Input: part model. Units: mm. Frame: model coordinates. Round coordinates to 2 decimals unless told otherwise and drop trailing zeros. Loops run counter-clockwise (first coordinate to the right, second up) from the corner with the lowest first, then second, coordinate; pieces in that order, holes last. Notation, with made-up numbers: M -33,16 L 8,16 A15 ccw 8,25 Z; hole C -4,69 d4. An arc over 180 degrees is marked long. Put each result on its own line as item: value. Start each with the question number.
1) Section B-B on z = 0.25. State how many separate pieces and enclosed holes the cut face has, plus the area to 3 significant figures.
2) Line query: probe 1 along X at (y, z) = (-4.75, 1.2); probe 2 along X at (y, z) = (-6.25, 0.3); probe 3 along Y at (x, z) = (18, 0.9) (3 decimals). Output: solid intervals per line, ascending.
3) Section A-A on y = 5.5. Output: boundary loops of the cut face in (x, z), plus the area to 3 significant figures.
4) Pin query (flat end, axial travel): pin 1 (12 mm diameter, centred on x = 43.5, y = 5.5, fed in from -Z); pin 2 (3 mm diameter, centred on x = 14.29, y = -4.76, fed in from +Z) (3 decimals). Return the tip coordinate at first contact, or that it passes through.
5) Section C-C on x = 19. Output: boundary loops of the cut face in (y, z) (1 decimal).
from build123d import *

# Parameters (mm, degrees)
F0_R     = 1.7272
F1_DEPTH = 1.5875


with BuildPart() as f1:
    # F0 (on Top) → F1 (new body)
    with BuildSketch(Plane.XY):
        with BuildLine():
            Line((0, 0), (0, -9.525))
            Line((0, -9.525), (55.515764, -9.525))
            Line((55.515764, -9.525), (55.515764, 0))
            Line((55.515764, 0), (30.030001, 11.420443))
            ThreePointArc((30.030001, 11.420443), (27.757882, 11.90625), (25.485763, 11.420443))
            Line((25.485763, 11.420443), (0, 0))
        make_face()
        with Locations((14.2875, -4.7625)):
            Circle(F0_R, mode=Mode.SUBTRACT)
        with Locations((41.228264, -4.7625)):
            Circle(F0_R, mode=Mode.SUBTRACT)
        with Locations((27.757882, 6.35)):
            Circle(F0_R, mode=Mode.SUBTRACT)
    extrude(amount=F1_DEPTH)


solid = f1.part
Geometry results:
1. separate pieces: 1
1. enclosed holes: 3
1. area: 845 mm²
2. probe 1: x = 0 to 12.56, 16.01 to 39.5, 42.96 to 55.52
2. probe 2: x = 0 to 13.41, 15.17 to 40.35, 42.11 to 55.52
2. probe 3: y = -9.525 to 8.066
3. outline: M 12.27,0 L 26.25,0 L 26.25,1.59 L 12.27,1.59 Z; M 29.26,0 L 43.24,0 L 43.24,1.59 L 29.26,1.59 Z
3. area: 44.4 mm²
4. pin 1: stops at z = 0
4. pin 2: passes through
5. outline: M -9.5,0 L 8.5,0 L 8.5,1.6 L -9.5,1.6 Z
